CAD build for the part. Positions are in the model's coordinates, mm. Face numbers are marked on the shaded views. A direction names the side the tool comes from. Round coordinates to 2 decimals unless told otherwise and drop trailing zeros. Order: outer loops, then holes, each group sorted by start corner. A loop starts at its lowest first (then second) coordinate and runs counter-clockwise, first axis right, second up. Notation, with made-up numbers: M 12,62 L 24,62 A13 ccw 24,80 Z; hole C 50.5,-23.5 d2. An arc over 180 degrees is marked long. Put each result on its own line as item: value.
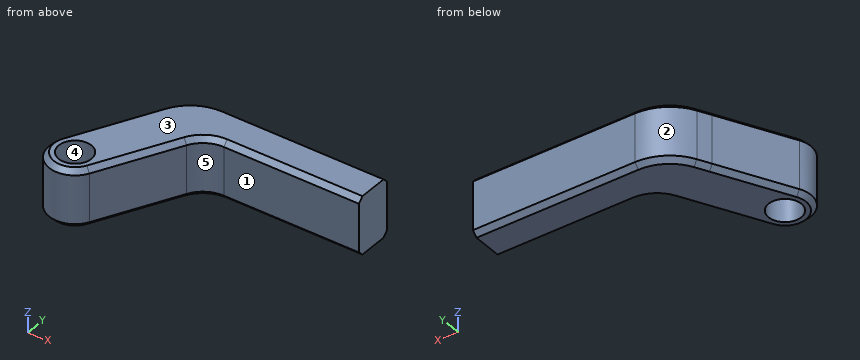
```python
from build123d import *

# Parameters (mm, degrees)
SKETCH1_R           = 5.375
SKETCH1_R_2         = 3.375
BOSS_EXTRUDE1_DEPTH = 12
FILLET1_R           = 10
FILLET1_2_R         = 6
CHAMFER1_SIZE       = 1


with BuildPart() as part:
    # Sketch1 → Boss-Extrude1 (new body)
    with BuildSketch(Plane.XY):
        Circle(SKETCH1_R)
        Circle(SKETCH1_R_2, mode=Mode.SUBTRACT)
        with BuildLine():
            Line((14.806897165, 17), (2.713546265, 17))
            Line((2.713546265, 17), (-4.777935452, 2.462104347))
            ThreePointArc((-4.777935452, 2.462104347), (1.2667324, 5.223601634), (5.375, 0))
            ThreePointArc((5.375, 0), (5.223601634, -1.2667324), (4.777935452, -2.462104347))
            Line((4.777935452, -2.462104347), (14.806897165, 17))
        make_face()
        Polygon((18.929354443, 25), (6.836003543, 25), (2.713546265, 17), (14.806897165, 17), align=None)
        Polygon((46.473934517, 25), (18.929354443, 25), (14.806897165, 17), (46.473934517, 17), align=None)
    extrude(amount=BOSS_EXTRUDE1_DEPTH)

    # Fillet1
    fillet1_edges = [part.edges().sort_by_distance(p)[0] for p in [
        (6.836003543, 25, 6),
    ]]
    fillet(fillet1_edges, radius=FILLET1_R)

    # Fillet1 2
    fillet1_2_edges = [part.edges().sort_by_distance(p)[0] for p in [
        (14.806897165, 17, 6),
    ]]
    fillet(fillet1_2_edges, radius=FILLET1_2_R)

    # Chamfer1
    chamfer1_edges = [part.edges().sort_by_distance(p)[0] for p in [
        (-2.462104347, -4.777935452, 12),
        (-2.462104347, -4.777935452, 0),
        (32.469382985, 17, 12),
        (8.954628782, 5.643145602, 0),
        (8.954628782, 5.643145602, 12),
        (-0.367278499, 11.021381799, 0),
        (-0.367278499, 11.021381799, 12),
        (29.703247603, 25, 0),
        (7.727111262, 23.538342711, 0),
        (29.703247603, 25, 12),
        (7.727111262, 23.538342711, 12),
        (15.341561797, 16.123005627, 0),
        (15.341561797, 16.123005627, 12),
        (32.469382985, 17, 0),
    ]]
    chamfer(chamfer1_edges, length=CHAMFER1_SIZE)


solid = part.part
```
Item 1: Band-saw the part on C-C on y = 0. Give the cut face in (x, z) (3 decimals), and give its area (3 significant figures).
Answers below:
outline: M -5.375,1 L -4.375,0 L -3.375,0 L -3.375,12 L -4.375,12 L -5.375,11 Z; M 3.375,0 L 4.922,0 L 6.047,1 L 6.047,11 L 4.922,12 L 3.375,12 Z
area: 53.9 mm²
Item 2: Band-saw the part on B-B on x = 0. Give the cut face in (y, z) (3 decimals), and give its area (3 significant figures).
Answers below:
outline: M -5.375,1 L -4.375,0 L -3.375,0 L -3.375,12 L -4.375,12 L -5.375,11 Z; M 3.375,0 L 9.551,0 L 11.734,1 L 11.734,11 L 9.551,12 L 3.375,12 Z
area: 121 mm²
Item 3: Pin check, flat tips, straight feed: P1, Ø2, axis at y = 3.5, z = 9.5, coming from the -X side; P2, Ø1.5, axis at y = 7.5, z = 8, coming from the +X side; P3, Ø2, axis at y = 8.5, z = 8.5, coming from the -X side. Stop position of each tip, or through.
Answers below:
P1: x = -4.76
P2: x = 10.3
P3: x = -2.18
Item 4: Probe line 1 along Y through (x, z) = (0, 9.25) (3 decimals); line 2 along X through (y, z) = (-1.5, 6.25); line 3 along Y through (x, z) = (43, 8.75). List the from-to ranges inside material, lowest first. Write a range as [from, to].
Answers below:
line 1: [-5.375, -3.375], [3.375, 11.734]
line 2: [-5.16, -3.02], [3.02, 5.27]
line 3: [17, 25]
Item 5: Band-saw the part on D-D on x = 25. Give the cut face in (y, z).
Answers below:
outline: M 17,1 L 18,0 L 24,0 L 25,1 L 25,11 L 24,12 L 18,12 L 17,11 Z
Item 6: Mould opens along Y. For the marked faces 3, 4 and 5 say: pulls with the +Y half, pulls with the -Y half, needs draft (parallel to the pull), parting line crosses it, or undercut.
Answers below:
face 3: needs draft
face 4: undercut
face 5: pulls with the -Y half
Item 7: Tool access for the marked faces 1 and 2: list every direction of +Z, -Z, +X, -X, +Y, -Y with a clear straight run to the whole face (end or side of a thin tool).
Answers below:
face 1: +Z, -Z, +X, -Y
face 2: +Z, -Z, -X, +Y
Item 8: Band-saw the part on A-A on z = 6. Give the cut face in (x, y) (3 decimals), and give its area (3 significant figures).
Answers below:
outline: M -4.778,2.462 A5.375 ccw 4.778,-2.462 L 13.131,13.748 A6 cw 18.465,17 L 46.474,17 L 46.474,25 L 12.933,25 A10 ccw 4.043,19.581 Z; hole C 0,0 d6.75
area: 545 mm²
